Build history of the part. All positions in model axes, mm. Give positions to 0.01 mm unless a question says otherwise; leave off trailing zeros. Write each loop counter-clockwise with the first axis right and the second up, starting at its lowest first coordinate (ties: lowest second). Pieces come first, ordered by that corner, then holes.
from build123d import *

# Parameters (mm, degrees)
ESBO_O1_W                = 43
ESBO_O1_H                = 135
RESSALTO_EXTRUS_O1_DEPTH = 21
ESBO_O2_W                = 4
ESBO_O2_H                = 8
RESSALTO_EXTRUS_O2_DEPTH = 21
FILETE2_R                = 3
FILETE3_R                = 3


with BuildPart() as part:
    # Esboço1 → Ressalto-extrusão1 (new body)
    with BuildSketch(Plane.XY):
        with Locations((21.5, 67.5)):
            Rectangle(ESBO_O1_W, ESBO_O1_H)
    extrude(amount=RESSALTO_EXTRUS_O1_DEPTH)

    # Esboço2 → Ressalto-extrusão2 (add)
    with BuildSketch(Plane(origin=(0, 135, 0), x_dir=(1, 0, 0), z_dir=(0, 1, 0))):
        with Locations((2, -4)):
            Rectangle(ESBO_O2_W, ESBO_O2_H)
    extrude(amount=RESSALTO_EXTRUS_O2_DEPTH)

    # Filete2
    filete2_edges = [part.edges().sort_by_distance(p)[0] for p in [
        (43, 67.5, 21),
        (0, 67.5, 21),
        (43, 67.5, 0),
        (21.5, 0, 0),
        (0, 78, 0),
        (43, 0, 10.5),
        (0, 0, 10.5),
        (21.5, 0, 21),
    ]]
    fillet(filete2_edges, radius=FILETE2_R)

    # Filete3
    filete3_edges = [part.edges().sort_by_distance(p)[0] for p in [
        (0, 135, 13),
        (21.5, 135, 21),
        (43, 135, 10.5),
        (22, 135, 0),
        (42.121320344, 135, 20.121320344),
        (0.878679656, 135, 20.121320344),
        (42.121320344, 135, 0.878679656),
    ]]
    fillet(filete3_edges, radius=FILETE3_R)


solid = part.part
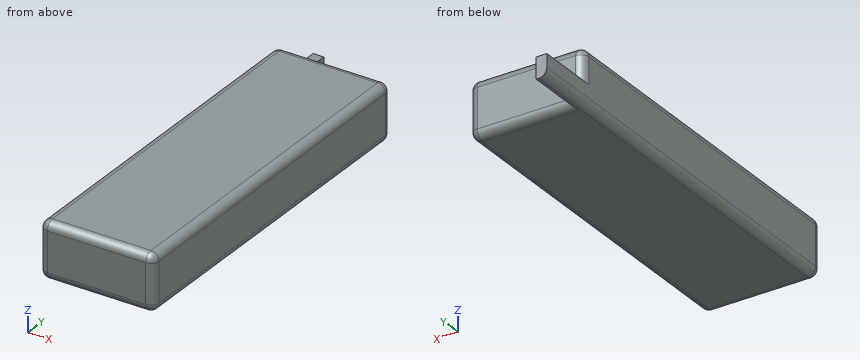
(1) Probe line 1 (Y direction, x = 29.5, z = 14.5); line 2 (X direction, y = 18.5, z = 1.5); line 3 (Y direction, x = 21.5, z = 19). List the from-to ranges inside material, lowest first.
(2) Saw through at A-A, the plane z = 13. List the corners of the cut face in (x, y).
(3) Drop flat-ended pins along their axis: pin 1 (4 mm diameter, centred on x = 13.5, z = 5, fed in from +Y); pin 2 (2 mm diameter, centred on x = 2.5, y = 145, fed in from +Z); pin 3 (9 mm diameter, centred on y = 140.5, z = 5, fed in from +X). Give the stop position or say it passes through.
(4) Saw through at C-C, the plane z = 4.75. List the corners of the cut face in (x, y).
(5) Saw through at B-B, the plane x = 12. List the corners of the cut face in (y, z).
Computed values:
1. line 1: y = 0 to 135
1. line 2: x = 0.4 to 42.6
1. line 3: y = 0.17 to 134.83
2. outline: (0, 3) arc R3 ccw to (3, 0) - (40, 0) arc R3 ccw to (43, 3) - (43, 132) arc R3 ccw to (40, 135) - (3, 135) arc R3 ccw to (0, 132) - close
3. pin 1: stops at y = 135
3. pin 2: stops at z = 8
3. pin 3: stops at x = 4
4. outline: (0, 3) arc R3 ccw to (3, 0) - (40, 0) arc R3 ccw to (43, 3) - (43, 132) arc R3 ccw to (40, 135) - (4, 135) - (4, 156) - (0, 156) - close
5. outline: (0, 3) arc R3 ccw to (3, 0) - (132, 0) arc R3 ccw to (135, 3) - (135, 18) arc R3 ccw to (132, 21) - (3, 21) arc R3 ccw to (0, 18) - close
